```python
from build123d import *

# Parameters (mm, degrees)
SKETCH1_W                        = 203.2
SKETCH1_H                        = 203.2
BOSS_EXTRUDE1_DEPTH              = 4.064
F_1_8_0_125_DIAMETER_HOLE1_D     = 3.175
F_1_8_0_125_DIAMETER_HOLE1_DEPTH = 25.4
F_1_8_0_125_DIAMETER_HOLE1_TIP   = 0.953866233
F_5_8_0_625_DIAMETER_HOLE1_D     = 31.75
F_5_8_0_625_DIAMETER_HOLE1_DEPTH = 25.4
F_5_8_0_625_DIAMETER_HOLE1_TIP   = 9.538662327


with BuildPart() as part:
    # Sketch1 → Boss-Extrude1 (new body)
    with BuildSketch(Plane(origin=(0, 0, 0), x_dir=(1, 0, 0), z_dir=(0, 1, 0))):
        Rectangle(SKETCH1_W, SKETCH1_H)
    extrude(amount=BOSS_EXTRUDE1_DEPTH)

    # 1/8 (0.125) Diameter Hole1
    with Locations(Plane(origin=(0, 4.064, 0), x_dir=(1, 0, 0), z_dir=(0, 1, 0))):
        with Locations((-83.82, 4.1275), (-58.42, 4.1275), (-58.42, -4.1275), (-83.82, -4.1275), (-4.1275, -83.82), (-4.1275, -58.42), (4.1275, -58.42), (4.1275, -83.82)):
            Hole(F_1_8_0_125_DIAMETER_HOLE1_D / 2, depth=F_1_8_0_125_DIAMETER_HOLE1_DEPTH)
            with Locations((0, 0, -(F_1_8_0_125_DIAMETER_HOLE1_DEPTH + F_1_8_0_125_DIAMETER_HOLE1_TIP / 2))):  # 118° drill point
                Cone(0, F_1_8_0_125_DIAMETER_HOLE1_D / 2, F_1_8_0_125_DIAMETER_HOLE1_TIP, mode=Mode.SUBTRACT)

    # 5/8 (0.625) Diameter Hole1
    with Locations(Plane(origin=(0, 4.064, 0), x_dir=(1, 0, 0), z_dir=(0, 1, 0))):
        with Locations((0, 0)):
            Hole(F_5_8_0_625_DIAMETER_HOLE1_D / 2, depth=F_5_8_0_625_DIAMETER_HOLE1_DEPTH)
            with Locations((0, 0, -(F_5_8_0_625_DIAMETER_HOLE1_DEPTH + F_5_8_0_625_DIAMETER_HOLE1_TIP / 2))):  # 118° drill point
                Cone(0, F_5_8_0_625_DIAMETER_HOLE1_D / 2, F_5_8_0_625_DIAMETER_HOLE1_TIP, mode=Mode.SUBTRACT)


solid = part.part
```
The listing builds one solid part. Answer for the finished solid, in the listing's coordinates (mm). Round coordinates to 2 decimals unless told otherwise and drop trailing zeros. Loops run counter-clockwise (first coordinate to the right, second up) from the corner with the lowest first, then second, coordinate; pieces in that order, holes last.
Q1. Find the intervals of material crossed by line 1 (Z direction, x = -58.42, y = 2.75) (3 decimals); line 2 (Z direction, x = 6, y = 3.6), in increasing order.
Q2. For a pull along Z with two mould halves and no side action, classify faces 1 (the face through (21, 4.064, -1)), 2 (the face through (3.441, 2.004, 15.497)) as released by +Z, released by -Z, zero draft, split by the parting line, or undercut.
Q3. Section B-B, the plane z = 0 is taken. Determine the outline of the cut face in (x, y) (3 decimals).
Q4. Section C-C, the plane y = 2.9 is taken. Count the separate pieces of the cut face and the enclosed holes in it, then the cut area to 3 significant figures.
Q5. Section A-A, the plane x = 0 is taken. Determine the outline of the cut face in (y, z) (3 decimals).
Completed:
1. line 1: z = -101.6 to -5.715, -2.54 to 2.54, 5.715 to 101.6
1. line 2: z = -101.6 to -14.7, 14.7 to 101.6
2. face 1: zero draft
2. face 2: undercut
3. outline: (-101.6, 0) - (-15.875, 0) - (-15.875, 4.064) - (-101.6, 4.064) - close; (15.875, 0) - (101.6, 0) - (101.6, 4.064) - (15.875, 4.064) - close
4. separate pieces: 1
4. enclosed holes: 9
4. area: 40,400 mm2
5. outline: (0, -101.6) - (4.064, -101.6) - (4.064, -15.875) - (0, -15.875) - close; (0, 15.875) - (4.064, 15.875) - (4.064, 101.6) - (0, 101.6) - close
